Can you work these out from the model? Positions are in its coordinate system, mm. A direction names the side the tool comes from. Round coordinates to 2 decimals unless told otherwise and drop trailing zeros. Loops run counter-clockwise (first coordinate to the right, second up) from the corner with the lowest first, then second, coordinate; pieces in that order, holes last. Notation, with made-up numbers: M 14,-24.75 L 57,-24.75 A21 ccw 57,-10.75 Z; hole C -9.75,19 d2. An arc over 180 degrees is marked long. Return JSON: item names as keys, results as strings.
```python
from build123d import *

# Parameters (mm, degrees)
SKETCH1_W               = 82.55
SKETCH1_H               = 57.15
BOSS_EXTRUDE1_DEPTH     = 20.32
FILLET2_R               = 7.62
FILLET3_R               = 3.81
SKETCH2_W               = 63.5
SKETCH2_H               = 40.64
CUT_EXTRUDE1_DEPTH      = 17.78
SKETCH9_W               = 15.46152766
SKETCH9_H               = 16.51
BOSS_EXTRUDE5_DEPTH     = 5.08
FILLET10_R              = 7.62
SKETCH7_W               = 71.12
SKETCH7_H               = 48.26
CUT_EXTRUDE4_DEPTH      = 5.461
FILLET12_R              = 2.54
FILLET13_R              = 1.27
SKETCH5_R               = 3.175
BOSS_EXTRUDE6_DEPTH     = 17.78
SKETCH11_R              = 1.27
CUT_EXTRUDE5_DEPTH      = 17.78
CUT_EXTRUDE_THIN1_DEPTH = 102.964471319


with BuildPart() as part:
    # Sketch1 → Boss-Extrude1 (new body)
    with BuildSketch(Plane(origin=(0, 0, 0), x_dir=(1, 0, 0), z_dir=(0, 1, 0))):
        with Locations((41.275, 28.575)):
            Rectangle(SKETCH1_W, SKETCH1_H)
    extrude(amount=BOSS_EXTRUDE1_DEPTH)

    # Fillet2
    fillet2_edges = [part.edges().sort_by_distance(p)[0] for p in [
        (0, 10.16, -57.15),
        (82.55, 10.16, -57.15),
        (82.55, 10.16, 0),
        (0, 10.16, 0),
    ]]
    fillet(fillet2_edges, radius=FILLET2_R)

    # Fillet3
    fillet3_edges = [part.edges().sort_by_distance(p)[0] for p in [
        (41.275, 0, -57.15),
        (0, 0, -28.575),
        (82.55, 0, -28.575),
        (41.275, 0, 0),
        (2.231846327, 0, -54.918153673),
        (2.231846327, 0, -2.231846327),
        (80.318153673, 0, -2.231846327),
        (80.318153673, 0, -54.918153673),
    ]]
    fillet(fillet3_edges, radius=FILLET3_R)

    # Sketch2 → Cut-Extrude1 (cut)
    with BuildSketch(Plane(origin=(0, 20.32, 0), x_dir=(1, 0, 0), z_dir=(0, 1, 0))):
        with Locations((41.275, 28.575)):
            Rectangle(SKETCH2_W, SKETCH2_H)
    extrude(amount=-CUT_EXTRUDE1_DEPTH, mode=Mode.SUBTRACT)

    # Sketch9 → Boss-Extrude5 (add)
    with BuildSketch(Plane.XY):
        with Locations((41.275, 12.065)):
            Rectangle(SKETCH9_W, SKETCH9_H)
    extrude(amount=BOSS_EXTRUDE5_DEPTH)

    # Fillet10
    # the kernel refuses this fillet: 7.62 mm, written as the material it takes off along each edge
    with BuildSketch(Plane(origin=(49.00576383, -14.150512242, 5.08), x_dir=(-1, 0, 0), z_dir=(0, 1, 0))) as fillet10_piece_1:
        with BuildLine():
            CenterArc((7.184204897, -7.62), FILLET10_R, 90, 70.528779366)
            Line((0, -5.08), (-0.143684098, -5.0292))
            ThreePointArc((-0.143684098, -5.0292), (-0.1524, -2.54), (-0.1524, 0))
            Line((-0.1524, 0), (0, 0.1524))
            Line((0, 0.1524), (7.184204897, 0.1524))
            Line((7.184204897, 0.1524), (7.184204897, 0))
        make_face()
    extrude(amount=52.431024484, mode=Mode.SUBTRACT)
    with BuildSketch(Plane(origin=(33.54423617, 38.280512242, 5.08), x_dir=(0, 0, -1), z_dir=(0, -1, 0))) as fillet10_piece_2:
        with BuildLine():
            CenterArc((7.62, 7.184204897), FILLET10_R, 180, 70.528779366)
            Line((0, 7.184204897), (-0.1524, 7.184204897))
            Line((-0.1524, 7.184204897), (-0.1524, 0))
            Line((-0.1524, 0), (0, -0.1524))
            ThreePointArc((0, -0.1524), (2.54, -0.1524), (5.0292, -0.143684098))
            Line((5.0292, -0.143684098), (5.08, 0))
        make_face()
    extrude(amount=52.431024484, mode=Mode.SUBTRACT)

    # Sketch7 → Cut-Extrude4 (cut)
    with BuildSketch(Plane(origin=(0, 20.32, 0), x_dir=(1, 0, 0), z_dir=(0, 1, 0))):
        with Locations((41.275, 28.575)):
            Rectangle(SKETCH7_W, SKETCH7_H)
    extrude(amount=-CUT_EXTRUDE4_DEPTH, mode=Mode.SUBTRACT)

    # Fillet12
    fillet12_edges = [part.edges().sort_by_distance(p)[0] for p in [
        (5.715, 17.5895, -52.705),
        (76.835, 17.5895, -52.705),
        (76.835, 17.5895, -4.445),
        (5.715, 17.5895, -4.445),
    ]]
    fillet(fillet12_edges, radius=FILLET12_R)

    # Fillet13
    fillet13_edges = [part.edges().sort_by_distance(p)[0] for p in [
        (41.275, 20.32, -52.705),
        (76.835, 20.32, -28.575),
        (41.275, 20.32, -4.445),
        (5.715, 20.32, -28.575),
        (76.091051224, 20.32, -51.961051224),
        (76.091051224, 20.32, -5.188948776),
        (6.458948776, 20.32, -51.961051224),
        (6.458948776, 20.32, -5.188948776),
    ]]
    fillet(fillet13_edges, radius=FILLET13_R)

    # Sketch5 → Boss-Extrude6 (add)
    with BuildSketch(Plane(origin=(0, 2.54, 0), x_dir=(1, 0, 0), z_dir=(0, 1, 0))):
        with Locations(Location((14.605, 42.291, 0), (0, 0, 90))):
            Circle(SKETCH5_R)
        with Locations(Location((14.605, 14.859, 0), (0, 0, 90))):
            Circle(SKETCH5_R)
        with Locations(Location((64.897, 42.291, 0), (0, 0, 90))):
            Circle(SKETCH5_R)
        with Locations(Location((64.896358582, 14.605, 0), (0, 0, 90))):
            Circle(SKETCH5_R)
    extrude(amount=BOSS_EXTRUDE6_DEPTH)

    # Sketch11 → Cut-Extrude5 (cut)
    with BuildSketch(Plane(origin=(0, 20.32, 0), x_dir=(1, 0, 0), z_dir=(0, 1, 0))):
        with Locations(Location((14.605, 14.859, 0), (0, 0, 270))):
            Circle(SKETCH11_R)
        with Locations(Location((14.605, 42.291, 0), (0, 0, 270))):
            Circle(SKETCH11_R)
        with Locations(Location((64.896358582, 14.605, 0), (0, 0, 270))):
            Circle(SKETCH11_R)
        with Locations(Location((64.897, 42.291, 0), (0, 0, 270))):
            Circle(SKETCH11_R)
    extrude(amount=-CUT_EXTRUDE5_DEPTH, mode=Mode.SUBTRACT)

    # Sketch17 → Cut-Extrude-Thin1 (cut, through all)
    with BuildSketch(Plane(origin=(0, 2.54, 0), x_dir=(1, 0, 0), z_dir=(0, 1, 0))):
        with BuildLine():
            ThreePointArc((18.78, 42.291), (17.557170811, 39.338829189), (14.605, 38.116))
            Line((14.605, 38.116), (14.605, 41.656))
            ThreePointArc((14.605, 41.656), (15.054012806, 41.841987194), (15.24, 42.291))
            Line((15.24, 42.291), (18.78, 42.291))
        make_face()
        with BuildLine():
            ThreePointArc((60.721358582, 14.605), (61.94418777, 17.557170811), (64.896358582, 18.78))
            Line((64.896358582, 18.78), (64.896358582, 15.24))
            ThreePointArc((64.896358582, 15.24), (64.447345776, 15.054012806), (64.261358582, 14.605))
            Line((64.261358582, 14.605), (60.721358582, 14.605))
        make_face()
        with BuildLine():
            ThreePointArc((14.605, 19.034), (17.557170811, 17.811170811), (18.78, 14.859))
            Line((18.78, 14.859), (15.24, 14.859))
            ThreePointArc((15.24, 14.859), (15.054012806, 15.308012806), (14.605, 15.494))
            Line((14.605, 15.494), (14.605, 19.034))
        make_face()
        with BuildLine():
            ThreePointArc((64.627, 42.291), (64.706081169, 42.100081169), (64.897, 42.021))
            Line((64.897, 42.021), (64.897, 38.481))
            ThreePointArc((64.897, 38.481), (62.202923164, 39.596923164), (61.087, 42.291))
            Line((61.087, 42.291), (64.627, 42.291))
        make_face()
    extrude(amount=CUT_EXTRUDE_THIN1_DEPTH, mode=Mode.SUBTRACT)


solid = part.part
```
Q1. Suppose I cut it at A-A, the plane y = 6.5. State how many separate pieces and enclosed holes the cut face has, plus the area to 3 significant figures.
Results:
{"separate pieces": "5", "enclosed holes": "1", "area": "2,230 mm2"}
Q2. Suppose I cut it at B-B, the plane z = -29. Please give me the cut outline in (x, y) (3 decimals), plus the area to 3 significant figures.
Results:
{"outline": "M 0,3.81 A3.81 ccw 3.81,0 L 78.74,0 A3.81 ccw 82.55,3.81 L 82.55,20.32 L 78.105,20.32 A1.27 ccw 76.835,19.05 L 76.835,14.859 L 73.025,14.859 L 73.025,2.54 L 9.525,2.54 L 9.525,14.859 L 5.715,14.859 L 5.715,19.05 A1.27 ccw 4.445,20.32 L 0,20.32 Z", "area": "500 mm2"}
Q3. If I drill on line 1 along X through (y, z) = (13, -24.5) (3 decimals); line 2 along X through (y, z) = (12.25, -44.5) (3 decimals); line 3 along Z through (x, y) = (66, 9) (3 decimals), over which ranges is the centre line in solid material (lowest first)?
Results:
{"line 1": "x = 0 to 9.525, 73.025 to 82.55", "line 2": "x = 0 to 9.525, 12.324 to 16.886, 62.616 to 67.178, 73.025 to 82.55", "line 3": "z = -57.15 to -48.895, -45.268 to -42.921, -41.661 to -39.314, -17.582 to -15.233, -13.977 to -11.628, -8.255 to 0"}
Q4. Suppose I cut it at C-C, the plane x = 20. Please give me the cut outline in (y, z) (3 decimals).
Results:
{"outline": "M 0,-53.34 A3.81 ccw 3.81,-57.15 L 20.32,-57.15 L 20.32,-53.975 A1.27 ccw 19.05,-52.705 L 14.859,-52.705 L 14.859,-48.895 L 2.54,-48.895 L 2.54,-8.255 L 14.859,-8.255 L 14.859,-4.445 L 19.05,-4.445 A1.27 ccw 20.32,-3.175 L 20.32,0 L 3.81,0 A3.81 ccw 0,-3.81 Z"}
Q5. Suppose I cut it at D-D, the plane x = 48. Please give me the cut outline in (y, z) (3 decimals).
Results:
{"outline": "M 0,-53.34 A3.81 ccw 3.81,-57.15 L 20.32,-57.15 L 20.32,-53.975 A1.27 ccw 19.05,-52.705 L 14.859,-52.705 L 14.859,-48.895 L 2.54,-48.895 L 2.54,-8.255 L 14.859,-8.255 L 14.859,-4.445 L 19.05,-4.445 A1.27 ccw 20.32,-3.175 L 20.32,1.92 L 3.81,1.92 L 3.81,0 A3.81 ccw 0,-3.81 Z"}
Q6. On a 3-axis mill with a long thin cutter (end or side, diameter ignored), from which of +Z, -Z, +X, -X, +Y, -Y can I reach the whole of each face in a straight line? I mean faces 1 (the flat face through (41, 9, -8.255)), 2 (the flat face through (66.3, 20.32, -13.9)). Say none if no direction works.
Results:
{"face 1": "+Y", "face 2": "+Z, -Z, +X, -X, +Y"}
Q7. Thinking about a two-plate mould opening in X: for faces 3 (the flat face through (15, 20.32, -13)), 4 (the flat face through (41, 2.54, -29)), 5 (the cylindrical face through (36.383, 12.181, 3.719)), which applies, pulls with the +X half, pulls with the -X half, needs draft (parallel to the pull), parting line crosses it, or undercut?
Results:
{"face 3": "needs draft", "face 4": "undercut", "face 5": "pulls with the -X half"}
Q8. I'm going to push flat-ended pins straight in: pin 1 Ø5 at (y, z) = (4.5, -6.5) entering from +X; pin 2 Ø1.5 at (y, z) = (2, -26) entering from +X; pin 3 Ø2.5 at (x, z) = (41.5, 3) entering from -Y; pin 4 Ø1.5 at (x, y) = (62.5, 11.5) entering from +Z. Where does each tip first touch, or does it pass through?
Results:
{"pin 1": "stops at x = 82.55", "pin 2": "stops at x = 82.4", "pin 3": "stops at y = 3.81", "pin 4": "stops at z = 0"}
